Check sheet for the drawn part. Datum: minimum x, y, z corner. Units: mm. A direction names the side the tool comes from. Give positions to 0.01 mm unless a question says otherwise; leave off trailing zeros. Write each loop counter-clockwise with the first axis right and the second up, starting at its lowest first coordinate (ties: lowest second). Pieces come first, ordered by that corner, then holes. Notation, with made-up numbers: M -14.5,60 L -3.5,60 A26 ccw -3.5,96 Z; hole C -17.5,83 d7. An arc over 180 degrees is marked long. Write item = value, one per line.
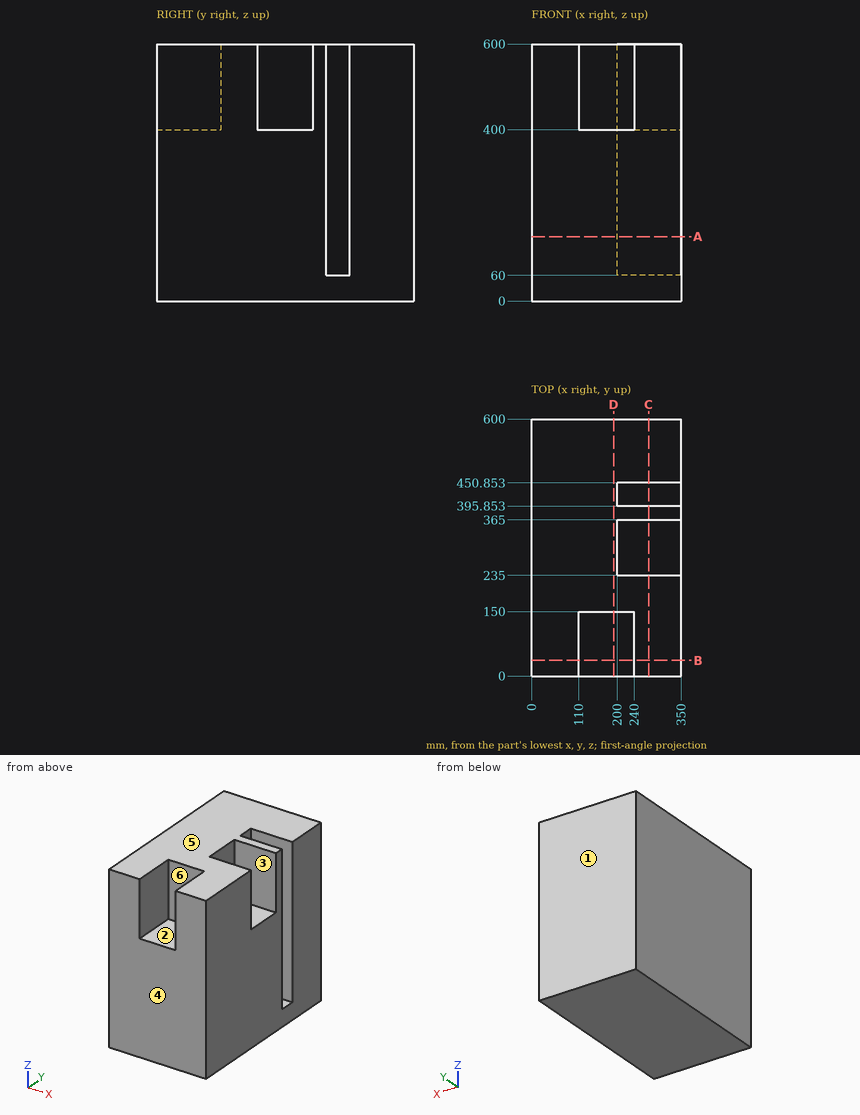
1) Tool access check on the marked faces 5 and 6. Record the directions out of +Z, -Z, +X, -X, +Y, -Y that give a thin tool (end or side, any length) a straight path to the whole face; none if there is none.
From the geometry:
face_5 = +Z, +X, -X, +Y, -Y
face_6 = +Z, -Y
2) Material ranges on probe 1 along X at (y, z) = (120, 455.5); probe 2 along Y at (x, z) = (236, 395.5); probe 3 along Y at (x, z) = (158.5, 415), recorded low to high. Write a range as from..to.
From the geometry:
probe_1 = 0..110, 240..350
probe_2 = 0..395.85, 450.85..600
probe_3 = 150..600
3) Cross-section at D-D on x = 191.5. Record the boundary of the cut face in (y, z).
From the geometry:
outline = M 0,0 L 600,0 L 600,600 L 150,600 L 150,400 L 0,400 Z
4) Draft check along Y on the marked faces 1, 2, 3 and 4. Enter one of: +Y half, -Y half, draft (parallel to the pull), parting line (faces both ways), or undercut.
From the geometry:
face_1 = +Y half
face_2 = draft
face_3 = undercut
face_4 = -Y half
5) Cross-section at C-C on x = 273.5. Record the boundary of the cut face in (y, z), plus the area to 3 significant figures.
From the geometry:
outline = M 0,0 L 600,0 L 600,600 L 450.85,600 L 450.85,60 L 395.85,60 L 395.85,600 L 365,600 L 365,400 L 235,400 L 235,600 L 0,600 Z
area = 304,000 mm^2
6) Depth check by flat-ended pin: P1, Ø16.5, axis at x = 276, y = 436, coming from the +Z side; P2, Ø5, axis at y = 263, z = 536.5, coming from the +X side. Enter the tip coordinate at first touch or a pass-through.
From the geometry:
P1 = 60
P2 = 200
7) Cross-section at B-B on y = 36.5. Record the boundary of the cut face in (x, z).
From the geometry:
outline = M 0,0 L 350,0 L 350,600 L 240,600 L 240,400 L 110,400 L 110,600 L 0,600 Z
8) Cross-section at A-A on z = 150. Record the boundary of the cut face in (x, y), plus the area to 3 significant figures.
From the geometry:
outline = M 0,0 L 350,0 L 350,395.85 L 200,395.85 L 200,450.85 L 350,450.85 L 350,600 L 0,600 Z
area = 202,000 mm^2
